Check sheet for the drawn part. Datum: minimum x, y, z corner. Units: mm. A direction names the side the tool comes from. Round coordinates to 2 decimals unless told otherwise and drop trailing zeros. Write each loop counter-clockwise with the first axis right and the second up, starting at its lowest first coordinate (ties: lowest second). Pieces come first, ordered by that corner, then holes. Notation, with made-up numbers: (-19.5, -2.5) -> (18.5, -2.5) arc R29 cw to (18.5, 22.5) -> close; hole circle Ø2 at (14.25, 66). An arc over 180 degrees is marked (long way). Use a Markdown table: item, result.
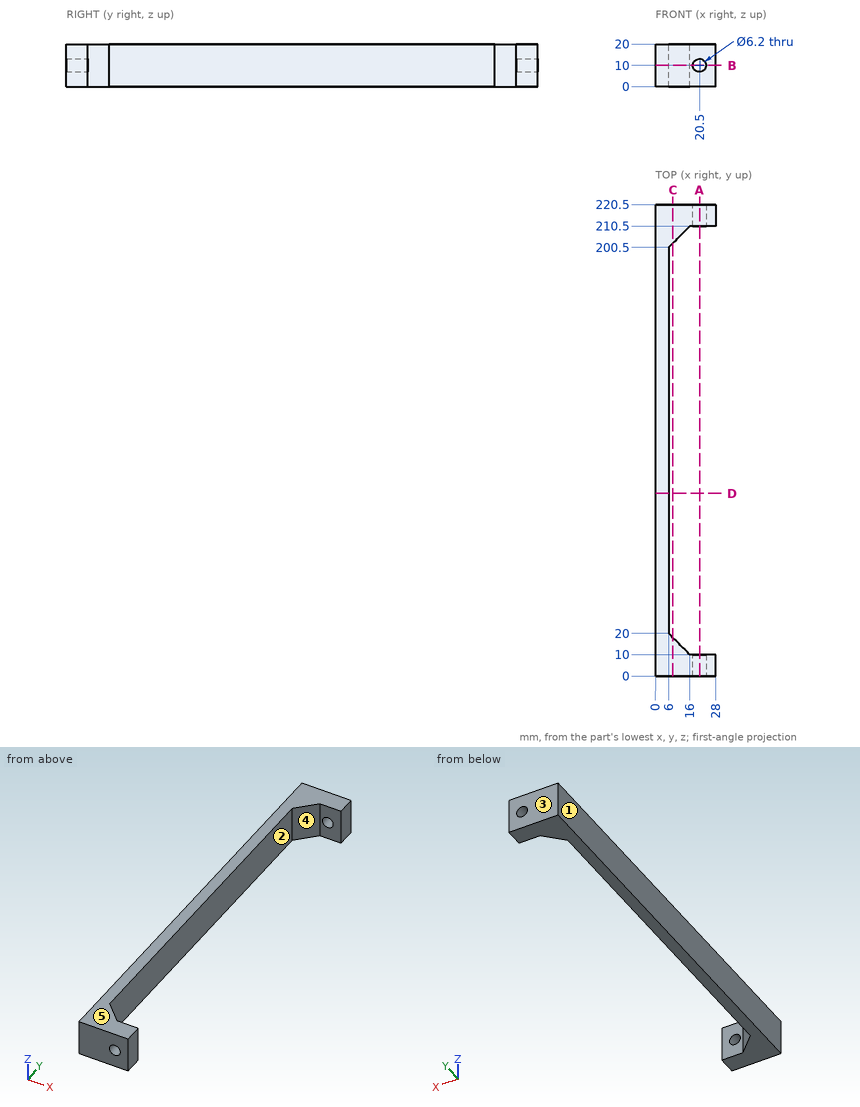
(1) Section check D-D on y = 85.5. Record the cut outline in (x, z), plus the area to 3 significant figures.
A:
| item | result |
|---|---|
| outline | (0, 0) -> (6, 0) -> (6, 20) -> (0, 20) -> close |
| area | 120 mm2 |
(2) Section check A-A on x = 20.5. Record the cut outline in (y, z).
A:
| item | result |
|---|---|
| outline | (0, 0) -> (10, 0) -> (10, 6.9) -> (0, 6.9) -> close; (0, 13.1) -> (10, 13.1) -> (10, 20) -> (0, 20) -> close; (210.5, 0) -> (220.5, 0) -> (220.5, 6.9) -> (210.5, 6.9) -> close; (210.5, 13.1) -> (220.5, 13.1) -> (220.5, 20) -> (210.5, 20) -> close |
(3) Access from +Z, -Z, +X, -X, +Y, -Y to the whole of each face (thin tool, end or side, straight path). Record for the marked faces 1 and 2.
A:
| item | result |
|---|---|
| face 1 | +Z, -Z, -X, +Y, -Y |
| face 2 | +Z, -Z, +X |
(4) Thickness scan on line 1 (Z direction, x = 20.5, y = 213.5); line 2 (Y direction, x = 19.75, z = 15.75); line 3 (X direction, y = 212.75, z = 10). Record the ranges inside material, lowest first.
A:
| item | result |
|---|---|
| line 1 | z = 0 to 6.9, 13.1 to 20 |
| line 2 | y = 0 to 10, 210.5 to 220.5 |
| line 3 | x = 0 to 17.4, 23.6 to 28 |
(5) Release check for a two-part mould opening along Y. For the marked faces 3, 4 and 5 record: +Y half, -Y half, draft (parallel to the pull), parting line (faces both ways), or undercut.
A:
| item | result |
|---|---|
| face 3 | +Y half |
| face 4 | undercut |
| face 5 | draft |
(6) Gauge pin test, flat end, axial feed: pin 1 Ø5 at (y, z) = (108.5, 3) entering from +X. Record the tip position at first contact, or that the pin passes through.
A:
| item | result |
|---|---|
| pin 1 | stops at x = 6 |
(7) Section check B-B on z = 10. Record the cut outline in (x, y), plus the area to 3 significant figures.
A:
| item | result |
|---|---|
| outline | (0, 0) -> (17.4, 0) -> (17.4, 10) -> (16, 10) -> (6, 20) -> (6, 200.5) -> (16, 210.5) -> (17.4, 210.5) -> (17.4, 220.5) -> (0, 220.5) -> close; (23.6, 0) -> (28, 0) -> (28, 10) -> (23.6, 10) -> close; (23.6, 210.5) -> (28, 210.5) -> (28, 220.5) -> (23.6, 220.5) -> close |
| area | 1,740 mm2 |
(8) Section check C-C on x = 8. Record the cut outline in (y, z), plus the area to 3 significant figures.
A:
| item | result |
|---|---|
| outline | (0, 0) -> (18, 0) -> (18, 20) -> (0, 20) -> close; (202.5, 0) -> (220.5, 0) -> (220.5, 20) -> (202.5, 20) -> close |
| area | 720 mm2 |
